For this review, take the finished solid that the model builds, in its own axes (mm). Coordinates: 2 decimals unless noted, no trailing zeros. Loops run counter-clockwise (first coordinate to the right, second up) from the corner with the lowest first, then second, coordinate; pieces in that order, holes last.
```python
from build123d import *

# Parameters (mm, degrees)
SKETCH1_R           = 22.5
SKETCH1_R_2         = 3.175
BOSS_EXTRUDE4_DEPTH = 6.35
FILLET1_R           = 78.74
FILLET3_R           = 3.175


with BuildPart() as part:
    # Sketch1 → Boss-Extrude4 (new body)
    with BuildSketch(Plane(origin=(0, 0, 0), x_dir=(1, 0, 0), z_dir=(0, 1, 0))):
        with BuildLine():
            ThreePointArc((-12.576911226, -43.956111111), (0, -58.42), (12.576911226, -43.956111111))
            ThreePointArc((12.576911226, -43.956111111), (24.319961907, -14.041136553), (44.355564487, 11.086130933))
            ThreePointArc((44.355564487, 11.086130933), (50.593204089, 29.21), (31.778653261, 32.869980178))
            ThreePointArc((31.778653261, 32.869980178), (0, 28.082273107), (-31.778653261, 32.869980178))
            ThreePointArc((-31.778653261, 32.869980178), (-50.593204089, 29.21), (-44.355564487, 11.086130933))
            ThreePointArc((-44.355564487, 11.086130933), (-24.319961907, -14.041136553), (-12.576911226, -43.956111111))
        make_face()
        Circle(SKETCH1_R, mode=Mode.SUBTRACT)
        with Locations((0, -45.72)):
            Circle(SKETCH1_R_2, mode=Mode.SUBTRACT)
        with Locations((-39.594681461, 22.86)):
            Circle(SKETCH1_R_2, mode=Mode.SUBTRACT)
        with Locations((39.594681461, 22.86)):
            Circle(SKETCH1_R_2, mode=Mode.SUBTRACT)
    extrude(amount=BOSS_EXTRUDE4_DEPTH)

    # Fillet1
    fillet1_edges = [part.edges().sort_by_distance(p)[0] for p in [
        (-12.576911226, 3.175, 43.956111111),
        (-44.355564487, 3.175, -11.086130933),
        (-31.778653261, 3.175, -32.869980178),
        (31.778653261, 3.175, -32.869980178),
        (44.355564487, 3.175, -11.086130933),
        (12.576911226, 3.175, 43.956111111),
    ]]
    fillet(fillet1_edges, radius=FILLET1_R)

    # Fillet3
    fillet3_edges = [part.edges().sort_by_distance(p)[0] for p in [
        (0, 6.35, -28.082273107),
        (50.593204089, 6.35, -29.21),
        (-50.593204089, 6.35, -29.21),
        (-24.319961907, 6.35, 14.041136554),
        (0, 6.35, 58.42),
        (24.319961907, 6.35, 14.041136553),
        (24.983104272, 6.35, -31.200471163),
        (-24.983104272, 6.35, -31.200471163),
        (-39.511952773, 6.35, -6.035767384),
        (-14.528848501, 6.35, 37.236238547),
        (14.528848501, 6.35, 37.236238547),
        (39.511952773, 6.35, -6.035767384),
    ]]
    fillet(fillet3_edges, radius=FILLET3_R)


solid = part.part
```
Q1. Consider section A-A (x = 0). State the section outline as (y, z) points (3 decimals).
Q2. Wall thickness on probe 1 along X at (y, z) = (2, -22.86); probe 2 along Z at (x, y) = (0, 2.25) (3 decimals); probe 3 along X at (y, z) = (4.5, -22.86): over which ranges is each line inside the solid? List them lowest first.
Q3. For pin 1 Ø5 at (x, z) = (-21.5, 31.5) entering from -Y; pin 2 Ø2 at (x, y) = (-36, 2.5) entering from +Z, all flat-tipped, find the tip position at first contact; note any pin that passes through.
Q4. The part is to be moulded in two halves that separate along X. For faces 1 (the face through (-24.4, 1.6, 13.9)), 2 (the face through (-22.1, 6.35, -5)), 3 (the face through (-0.41, 3.13, 42.57)), 4 (the face through (-42.767, 3.131, -23)), say which applies: +X half, -X half, draft (parallel to the pull), parting line (faces both ways), or undercut.
Q5. Consider section B-B (y = 1). Count the separate pieces of the cut face and the enclosed holes in it, then the cut area to 3 significant figures.
Model answer:
1. outline: (0, -28.082) - (3.175, -28.082) arc R3.175 ccw to (6.35, -24.907) - (6.35, -22.5) - (0, -22.5) - close; (0, 22.5) - (6.35, 22.5) - (6.35, 42.545) - (0, 42.545) - close; (0, 48.895) - (6.35, 48.895) - (6.35, 55.245) arc R3.175 ccw to (3.175, 58.42) - (0, 58.42) - close
2. probe 1: x = -52.29 to -42.77, -36.42 to 36.42, 42.77 to 52.29
2. probe 2: z = -28.082 to -22.5, 22.5 to 42.545, 48.895 to 58.42
2. probe 3: x = -52 to -42.77, -36.42 to 36.42, 42.77 to 52
3. pin 1: passes through
3. pin 2: stops at z = -1.2
4. face 1: -X half
4. face 2: draft
4. face 3: undercut
4. face 4: undercut
5. separate pieces: 1
5. enclosed holes: 4
5. area: 3,410 mm2
